Can you work these out from the model? Positions are in its coordinate system, mm. Face numbers are marked on the shaded views. A direction names the side the tool comes from. Round coordinates to 2 decimals unless told otherwise and drop trailing zeros. Loops run counter-clockwise (first coordinate to the right, second up) from the corner with the lowest first, then second, coordinate; pieces in that order, holes last.
```python
from build123d import *

# Parameters (mm, degrees)
SKETCH1_R           = 23.875
SKETCH1_R_2         = 16.875
BOSS_EXTRUDE1_DEPTH = 25
SKETCH2_W           = 25
SKETCH2_H           = 7
BOSS_EXTRUDE2_DEPTH = 75.83
BOSS_EXTRUDE3_DEPTH = 15
FILLET1_R           = 10
FILLET2_R           = 2
FILLET3_R           = 2
SKETCH5_W           = 21
SKETCH5_H           = 50
BOSS_EXTRUDE4_DEPTH = 3
CHAMFER1_SIZE       = 1


with BuildPart() as part:
    # Sketch1 → Boss-Extrude1 (new body)
    with BuildSketch(Plane(origin=(0, 0, 0), x_dir=(0, 0, -1), z_dir=(1, 0, 0))):
        Circle(SKETCH1_R)
        Circle(SKETCH1_R_2, mode=Mode.SUBTRACT)
    extrude(amount=BOSS_EXTRUDE1_DEPTH)

    # Sketch2 → Boss-Extrude2 (add)
    with BuildSketch(Plane(origin=(0, 0, 0), x_dir=(1, 0, 0), z_dir=(0, 1, 0))):
        with Locations((12.5, -20.375)):
            Rectangle(SKETCH2_W, SKETCH2_H)
    extrude(amount=BOSS_EXTRUDE2_DEPTH)

    # Sketch4 → Boss-Extrude3 (add)
    with BuildSketch(Plane.ZY.offset(-25)):
        with BuildLine():
            Line((-40.591185313, 40), (-48.125, 40))
            Line((-48.125, 40), (-48.125, 25))
            Line((-48.125, 25), (23.875, 25))
            Line((23.875, 25), (23.875, 75))
            Line((23.875, 75), (-48.125, 75))
            Line((-48.125, 75), (-48.125, 60))
            Line((-48.125, 60), (-40.591185313, 60))
            ThreePointArc((-40.591185313, 60), (-1.125, 50), (-40.591185313, 40))
        make_face()
    extrude(amount=BOSS_EXTRUDE3_DEPTH)

    # Fillet1
    fillet1_edges = [part.edges().sort_by_distance(p)[0] for p in [
        (17.5, 75, -48.125),
        (17.5, 25, -48.125),
    ]]
    fillet(fillet1_edges, radius=FILLET1_R)

    # Fillet2
    fillet2_edges = [part.edges().sort_by_distance(p)[0] for p in [
        (0, -9.141252649, -22.055682374),
        (0, 46.359672877, 16.875),
        (0, 37.915, 23.875),
        (0, 0, 16.875),
        (25, 0, 16.875),
    ]]
    fillet(fillet2_edges, radius=FILLET2_R)

    # Fillet3
    fillet3_edges = [part.edges().sort_by_distance(p)[0] for p in [
        (17.5, 60, -48.125),
        (17.5, 40, -48.125),
    ]]
    fillet(fillet3_edges, radius=FILLET3_R)

    # Sketch5 → Boss-Extrude4 (add)
    with BuildSketch(Plane.ZY.offset(-10)):
        with Locations((6.375, 50)):
            Rectangle(SKETCH5_W, SKETCH5_H)
    extrude(amount=BOSS_EXTRUDE4_DEPTH)

    # Chamfer1
    chamfer1_edges = [part.edges().sort_by_distance(p)[0] for p in [
        (7, 50, 16.875),
        (7, 50, -4.125),
    ]]
    chamfer(chamfer1_edges, length=CHAMFER1_SIZE)


solid = part.part
```
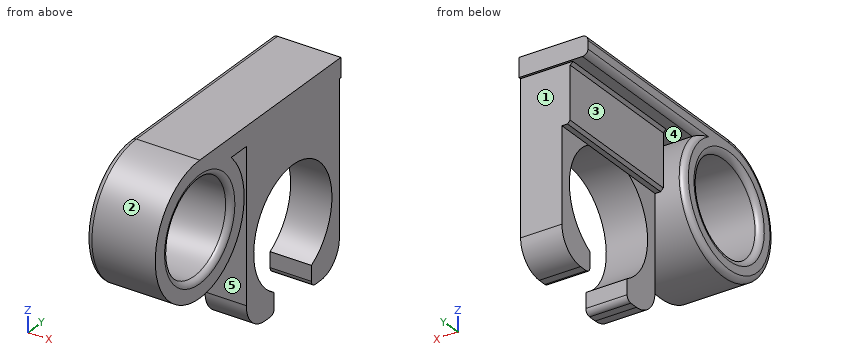
(1) Suppose I cut it at C-C (x = 21.5). Write out the boundary of the cut face in (y, z) (3 decimals), then the cut area to 3 significant figures.
(2) Suppose I cut it at A-A (z = 0). Write out the boundary of the cut face in (x, y) (3 decimals), then the cut area to 3 significant figures.
(3) Suppose I cut it at D-D (y = 50). Write out the boundary of the cut face in (x, z) (3 decimals).
(4) For pin 1 (6 mm diameter, centred on x = 18, z = 5.5, fed in from -Y); pin 2 (5.5 mm diameter, centred on y = 59, z = 2, fed in from -X); pin 3 (16.5 mm diameter, centred on y = 66.5, z = -18, fed in from -X); pin 4 (25 mm diameter, centred on y = 50, z = -22.125, fed in from +X), each with a flat end and sliding along its axis, tell me the tip position at first contact or that it passes through.
(5) If I drill on line 1 (Y direction, x = 15.75, z = 0) (3 decimals); line 2 (Y direction, x = 12.25, z = -7); line 3 (Y direction, x = 20.25, z = -9), over which ranges is the centre line in solid material (lowest first)?
(6) Suppose I cut it at B-B (z = -37). Write out the boundary of the cut face in (x, y).
(7) Which directions (+Z, -Z, +X, -X, +Y, -Y) give clear straight access to the entire face, cutting with the end or side of a thin tool? Please do the marked faces 1, 2, 3, 4 and 5.
Check result:
1. outline: (0, 23.875) arc R23.875 ccw (long way) to (16.889, 16.875) - (25, 16.875) - (25, -38.125) arc R10 ccw to (35, -48.125) - (38, -48.125) arc R2 ccw to (40, -46.125) - (40, -40.591) arc R21 cw (long way) to (60, -40.591) - (60, -46.125) arc R2 ccw to (62, -48.125) - (65, -48.125) arc R10 ccw to (75, -38.125) - (75, 16.875) - (75.83, 16.875) - (75.83, 23.875) - close; hole circle Ø33.75 at (0, 0)
1. area: 3,050 mm2
2. outline: (0, -21.875) arc R2 ccw to (2, -23.875) - (25, -23.875) - (25, -18.875) arc R2 ccw to (23, -16.875) - (2, -16.875) arc R2 ccw to (0, -18.875) - close; (0, 18.875) arc R2 ccw to (2, 16.875) - (23, 16.875) arc R2 ccw to (25, 18.875) - (25, 23.875) - (2, 23.875) arc R2 ccw to (0, 21.875) - close; (7, 25) - (25, 25) - (25, 75) - (7, 75) - close
2. area: 1,240 mm2
3. outline: (0, 18.875) arc R2 ccw to (2, 16.875) - (6, 16.875) - (7, 15.875) - (7, -3.125) - (8, -4.125) - (10, -4.125) - (10, -1.125) - (25, -1.125) - (25, 23.875) - (2, 23.875) arc R2 ccw to (0, 21.875) - close
4. pin 1: stops at y = -23.74
4. pin 2: stops at x = 7
4. pin 3: stops at x = 10
4. pin 4: passes through
5. line 1: y = -23.875 to -16.875, 16.875 to 23.875, 25 to 75
5. line 2: y = -22.83 to -15.35, 15.35 to 22.83, 25 to 35.43, 64.57 to 75
5. line 3: y = -22.11 to -14.27, 14.27 to 22.11, 25 to 33.61, 66.39 to 75
6. outline: (10, 25) - (25, 25) - (25, 35.18) - (10, 35.18) - close; (10, 64.82) - (25, 64.82) - (25, 75) - (10, 75) - close
7. face 1: -Z, +X, -X, +Y
7. face 2: +X, -X
7. face 3: -Z, -X, +Y
7. face 4: -X
7. face 5: -Z, +X, -X
